Autodesk Inventor part; units mm, degrees
ref_plane "YZ Plane" through (0, 0, 0) normal (1, 0, 0) x (0, 1, 0)
ref_plane "XZ Plane" through (0, 0, 0) normal (0, 1, 0) x (-1, 0, 0)
ref_plane "XY Plane" through (0, 0, 0) normal (0, 0, 1) x (1, 0, 0)
sketch "Sketch1" plane through (0, 0, 0) normal (0, 1, 0) x (-1, 0, 0)
  line L0 (-27, 20) -> (0, 20)
  line L1 (0, 20) -> (0, 0) construction
  line L2 (0, 0) -> (-27, 0) construction
  line L3 (-27, 0) -> (-27, 20)
  line L4 (-37.8717, 14) -> (4.6091, 14) construction
  circle A0 centre (-6, 14) radius 2
  circle A1 centre (-21, 14) radius 2
  line L5 (-27, -20) -> (0, -20)
  line L6 (0, -20) -> (0, 0) construction
  line L7 (-27, 0) -> (-27, -20)
  line L8 (-37.8717, -14) -> (4.6091, -14) construction
  circle A2 centre (-6, -14) radius 2
  circle A3 centre (-21, -14) radius 2
  line L9 (0, 20) -> (0, -20)
  dimension "d1" = 20
  dimension "d2" = 6
  dimension "d3" = 4
  dimension "d4" = 6
  dimension "d5" = 21
  dimension "d7" = 6
extrude "Plate1" add sketch "Sketch1" along normal blind 1
equation "\"BendRadius\" = Thickness"
equation "\"BendReliefWidth\" = Thickness"
equation "\"BendReliefDepth\" = 0.5 * Thickness"
equation "\"CornerReliefSize\" = 4 * Thickness"
equation "\"MinimumRemnant\" = 2 * Thickness"
equation "\"TransitionRadius\" = BendRadius"
equation "\"JacobiRadiusSize\" = BendRadius"
equation "\"GapSize\" = Thickness"
equation "\"d6\" = BendRadius"
properties part number "BracketHalf" material "Steel, Galvanized"
The model under review builds one solid part; all positions refer to its coordinate system, in mm. Round coordinates to 2 decimals unless told otherwise and drop trailing zeros. Loops run counter-clockwise (first coordinate to the right, second up) from the corner with the lowest first, then second, coordinate; pieces in that order, holes last. Notation, with made-up numbers: (-3, 73.25) -> (21, 73.25) arc R12 ccw to (21, 83.25) -> close; hole circle Ø11 at (-35, -32). An arc over 180 degrees is marked (long way). Return JSON: item names as keys, results as strings.
(1) For pin 1 (3.5 mm diameter, centred on x = 6, z = 14, fed in from -Y) (1 decimal), flat-tipped, find the tip position at first contact; note if it passes through.
Solved:
{"pin 1": "through"}
(2) Add section C-C on y = 0.4. Write out the cut boundary in (x, z), plus the area to 3 significant figures.
Solved:
{"outline": "(0, -20) -> (27, -20) -> (27, 20) -> (0, 20) -> close; hole circle Ø4 at (6, -14); hole circle Ø4 at (6, 14); hole circle Ø4 at (21, -14); hole circle Ø4 at (21, 14)", "area": "1,030 mm2"}
(3) Add section B-B on x = 21. Write out the cut boundary in (y, z), plus the area to 3 significant figures.
Solved:
{"outline": "(0, -20) -> (1, -20) -> (1, -16) -> (0, -16) -> close; (0, -12) -> (1, -12) -> (1, 12) -> (0, 12) -> close; (0, 16) -> (1, 16) -> (1, 20) -> (0, 20) -> close", "area": "32.0 mm2"}
(4) Add section A-A on z = -14. Write out the cut boundary in (x, y).
Solved:
{"outline": "(0, 0) -> (4, 0) -> (4, 1) -> (0, 1) -> close; (8, 0) -> (19, 0) -> (19, 1) -> (8, 1) -> close; (23, 0) -> (27, 0) -> (27, 1) -> (23, 1) -> close"}
(5) The part is to be moulded in two halves that separate along X. For faces 1 (the cylindrical face through (22.474, 0.493, -15.352)), 2 (the flat face through (13.7, 0.5, -20)), 3 (the flat face through (27, 0.5, 0.3)), say which applies: released by +X, released by -X, zero draft, split by the parting line, or undercut.
Solved:
{"face 1": "undercut", "face 2": "zero draft", "face 3": "released by +X"}
(6) For line 1 (Z direction, x = 6, y = 0.7); line 2 (X direction, y = 0.9, z = 13), list the stretches that pass through material, from the lowest coordinate up.
Solved:
{"line 1": "-20 to -16, -12 to 12, 16 to 20", "line 2": "0 to 4.27, 7.73 to 19.27, 22.73 to 27"}
